Design review of the part built by this model. Coordinates are the model's own, in mm. Face numbers are marked on the shaded views. A direction names the side the tool comes from. Coordinates: 2 decimals unless noted, no trailing zeros. Loops run counter-clockwise (first coordinate to the right, second up) from the corner with the lowest first, then second, coordinate; pieces in that order, holes last. Notation, with made-up numbers: (70.5, -5) -> (123.5, -5) arc R26 ccw to (123.5, 32) -> close; hole circle Ø7 at (-38.75, 35). An arc over 180 degrees is marked (long way). Use a Markdown table: item, result. Add a question column.
Q1. Clearance check with flat-ended pins moving along their axes: pin 1 Ø3 at (x, y) = (28, -28.5) entering from +Z; pin 2 Ø8 at (x, z) = (20.5, 96.5) entering from +Y. State where each tip first meets the part, or that it passes through.
Q2. Take a section at B-B on y = -49. Write out the cut boundary in (x, z), plus the area to 3 significant figures.
Q3. For the marked faces 5 and 6, list the 3-axis set-ups (+Z, -Z, +X, -X, +Y, -Y) from which the entire face can be reached by the end or side of a thin tool; tool diameter is ignored.
Q4. Take a section at A-A on x = 20. Write out the cut boundary in (y, z), plus the area to 3 significant figures.
Q5. For probe 1 along Z at (x, y) = (9.5, -47.5); probe 2 along Z at (x, y) = (58, -55.5); probe 3 along Z at (x, y) = (25.5, -11.5), list the stretches that pass through material, from the lowest coordinate up.
Q6. Take a section at C-C on x = 50. Write out the cut boundary in (y, z), plus the area to 3 significant figures.
Q7. Draft analysis for pull direction Z (two halves, no side actions). For the marked faces 1, 2, 3 and 4, state which applies: pulls with the +Z half, pulls with the -Z half, needs draft (parallel to the pull), parting line crosses it, or undercut.
Q8. Take a section at D-D on y = -68.5. Write out the cut boundary in (x, z).
from build123d import *

# Parameters (mm, degrees)
F0_W     = 89.99192
F0_H     = 59.686664
F1_DEPTH = 94.996
F2_R     = 25.458482
F3_DEPTH = 59.436
F4_W     = 58.544096
F4_H     = 15.645336
F5_DEPTH = 116.078


with BuildPart() as f1:
    # F0 (on Right) → F1 (new body)
    with BuildSketch(Plane.YZ):
        with Locations((-44.99596, 29.843332)):
            Rectangle(F0_W, F0_H)
    extrude(amount=F1_DEPTH)

    # F2 (on face) → F3 (join)
    with BuildSketch(Plane.XY.offset(59.686664)):
        with Locations((51.198136, -45.706607)):
            Circle(F2_R)
    extrude(amount=F3_DEPTH)

    # F4 (on face) → F5 (cut)
    with BuildSketch(Plane(origin=(0, 0, 0), x_dir=(0, -1, 0), z_dir=(-1, 0, 0))):
        with Locations((41.940892, 31.036956)):
            Rectangle(F4_W, F4_H)
    extrude(amount=-F5_DEPTH, mode=Mode.SUBTRACT)


solid = f1.part
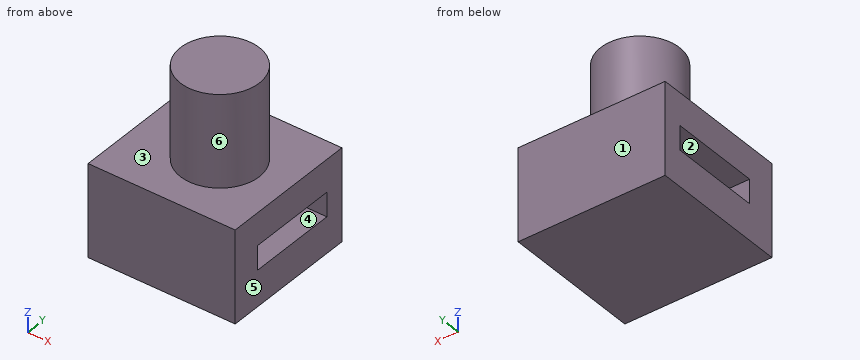
Answer list:
| question | item | result |
|---|---|---|
| 1 | pin 1 | z = 59.69 |
| 1 | pin 2 | through |
| 2 | outline | (0, 0) -> (95, 0) -> (95, 23.21) -> (0, 23.21) -> close; (0, 38.86) -> (95, 38.86) -> (95, 59.69) -> (76.44, 59.69) -> (76.44, 119.12) -> (25.95, 119.12) -> (25.95, 59.69) -> (0, 59.69) -> close |
| 2 | area | 7,180 mm² |
| 3 | face 5 | +Z, -Z, +X, +Y, -Y |
| 3 | face 6 | +Z |
| 4 | outline | (-89.99, 0) -> (0, 0) -> (0, 59.69) -> (-89.99, 59.69) -> close; hole (-71.21, 23.21) -> (-12.67, 23.21) -> (-12.67, 38.86) -> (-71.21, 38.86) -> close |
| 4 | area | 4,460 mm² |
| 5 | probe 1 | 0 to 23.21, 38.86 to 59.69 |
| 5 | probe 2 | 0 to 23.21, 38.86 to 119.12 |
| 5 | probe 3 | 0 to 59.69 |
| 6 | outline | (-89.99, 0) -> (0, 0) -> (0, 59.69) -> (-20.28, 59.69) -> (-20.28, 119.12) -> (-71.14, 119.12) -> (-71.14, 59.69) -> (-89.99, 59.69) -> close; hole (-71.21, 23.21) -> (-12.67, 23.21) -> (-12.67, 38.86) -> (-71.21, 38.86) -> close |
| 6 | area | 7,480 mm² |
| 7 | face 1 | needs draft |
| 7 | face 2 | undercut |
| 7 | face 3 | pulls with the +Z half |
| 7 | face 4 | undercut |
| 8 | outline | (0, 0) -> (95, 0) -> (95, 23.21) -> (0, 23.21) -> close; (0, 38.86) -> (95, 38.86) -> (95, 59.69) -> (62.54, 59.69) -> (62.54, 119.12) -> (39.86, 119.12) -> (39.86, 59.69) -> (0, 59.69) -> close |
